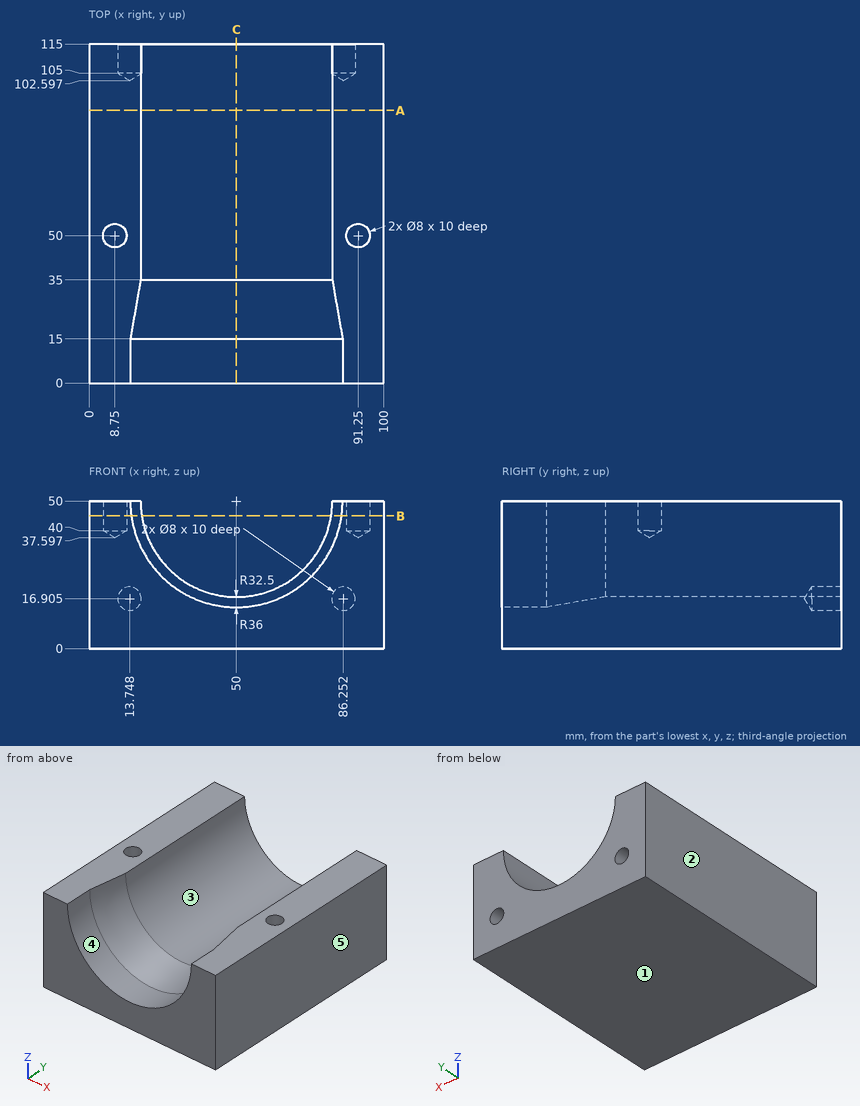
The drawing under review shows one solid part. Ordinate dimensions are in mm from its lowest x, y, z. A direction names the side the tool comes from. Coordinates: 2 decimals unless noted, no trailing zeros. Order: outer loops, then holes, each group sorted by start corner. A loop starts at its lowest first (then second) coordinate and runs counter-clockwise, first axis right, second up. Notation, with made-up numbers: (83.25, 6) -> (93.25, 6) arc R22 ccw to (93.25, 43) -> close; hole circle Ø7 at (70.5, 5.5). An arc over 180 degrees is marked (long way). Answer in a Markdown table with one row per item.
(1) The part is to be moulded in two halves that separate along X. For the marked faces 1, 2 and 3, say which applies: +X half, -X half, draft (parallel to the pull), parting line (faces both ways), or undercut.
Answers:
| item | result |
|---|---|
| face 1 | draft |
| face 2 | -X half |
| face 3 | undercut |
(2) Consider section B-B (z = 45). State how many separate pieces and enclosed holes the cut face has, plus the area to 3 significant figures.
Answers:
| item | result |
|---|---|
| separate pieces | 2 |
| enclosed holes | 2 |
| area | 3,840 mm² |
(3) Machinability: for the marked faces 4 and 5, which of the approach directions +Z, -Z, +X, -X, +Y, -Y give a long, thin tool a straight path to every point of the face, cutting with its end or side? Answer none if there is none.
Answers:
| item | result |
|---|---|
| face 4 | +Z, -Y |
| face 5 | +Z, -Z, +X, +Y, -Y |
(4) Wall thickness on line 1 along X through (y, z) = (50, 46); line 2 along X through (y, z) = (50, 45); line 3 along Y through (x, z) = (8.75, 43): over which ranges is each line inside the solid? List them lowest first.
Answers:
| item | result |
|---|---|
| line 1 | 0 to 4.75, 12.75 to 17.75, 82.25 to 87.25, 95.25 to 100 |
| line 2 | 0 to 4.75, 12.75 to 17.89, 82.11 to 87.25, 95.25 to 100 |
| line 3 | 0 to 46, 54 to 115 |
(5) Consider section A-A (y = 92.5). Write out the cut boundary in (x, z), plus the area to 3 significant figures.
Answers:
| item | result |
|---|---|
| outline | (0, 0) -> (100, 0) -> (100, 50) -> (82.5, 50) arc R32.5 cw to (17.5, 50) -> (0, 50) -> close |
| area | 3,340 mm² |
(6) Consider section C-C (x = 50). Write out the cut boundary in (y, z).
Answers:
| item | result |
|---|---|
| outline | (0, 0) -> (115, 0) -> (115, 17.5) -> (35, 17.5) -> (15, 14) -> (0, 14) -> close |
(7) Insertion check: pin 1 (5 mm diameter, centred on x = 8.75, y = 50, fed in from +Z); pin 2 (5 mm diameter, centred on x = 76.5, y = 19, fed in from +Z) (1 decimal). Each pin has a flat end and moves straight along its axis. Give the tip position at first contact, or say it passes through.
Answers:
| item | result |
|---|---|
| pin 1 | z = 39.1 |
| pin 2 | z = 30 |
